Input: part model. Units: mm. Frame: model coordinates. Face numbers are marked on the shaded views. A direction names the side the tool comes from. Round coordinates to 2 decimals unless told otherwise and drop trailing zeros. Order: outer loops, then holes, each group sorted by start corner. A loop starts at its lowest first (then second) coordinate and runs counter-clockwise, first axis right, second up. Notation, with made-up numbers: (-7.5, 34) -> (35.5, 34) arc R35 ccw to (35.5, 73) -> close; hole circle Ø1 at (79, 12.5). An arc over 180 degrees is marked (long way). Use a Markdown table: item, result.
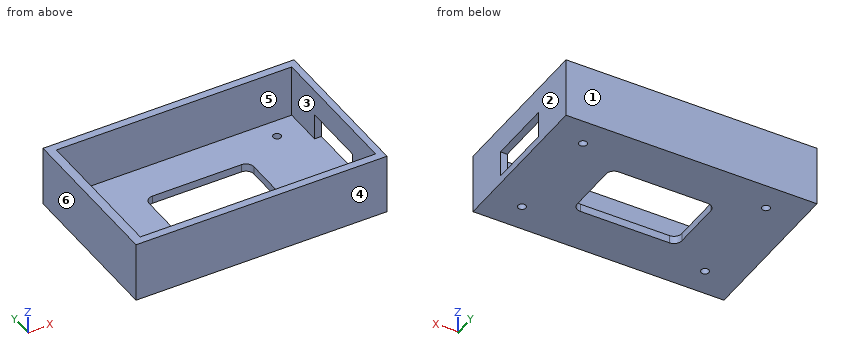
Autodesk Inventor part; units mm, degrees
ref_plane "YZ Plane" through (0, 0, 0) normal (1, 0, 0) x (0, 1, 0)
ref_plane "XZ Plane" through (0, 0, 0) normal (0, 1, 0) x (-1, 0, 0)
ref_plane "XY Plane" through (0, 0, 0) normal (0, 0, 1) x (1, 0, 0)
sketch "Sketch1" plane through (0, 0, 0) normal (0, 0, 1) x (1, 0, 0)
  line L0 (-50.0201, 33.5227) -> (45.9799, 33.5227)
  line L1 (45.9799, 33.5227) -> (45.9799, -27.4773)
  line L2 (45.9799, -27.4773) -> (-50.0201, -27.4773)
  line L3 (-50.0201, -27.4773) -> (-50.0201, 33.5227)
  line L4 (-50.0201, 33.5227) -> (-50.0201, 30.5227)
  line L5 (-46.6334, 30.5227) -> (43.3666, 30.5227)
  line L6 (43.3666, 30.5227) -> (43.3666, -24.4773)
  line L7 (43.3666, -24.4773) -> (-46.6334, -24.4773)
  line L8 (-46.6334, -24.4773) -> (-46.6334, 30.5227)
  circle A0 centre (-36.6334, 23.0227) radius 1.5
  circle A1 centre (33.3666, 23.0227) radius 1.5
  circle A2 centre (-36.6334, -16.9773) radius 1.5
  circle A3 centre (33.3666, -16.9773) radius 1.5
  line L9 (-18.6334, 15.5227) -> (15.3666, 15.5227)
  line L10 (18.3666, 12.5227) -> (18.3666, -6.4773)
  line L11 (15.3666, -9.4773) -> (-18.6334, -9.4773)
  line L12 (-21.6334, -6.4773) -> (-21.6334, 12.5227)
  arc A4 (-18.6334, 15.5227) -> (-21.6334, 12.5227) centre (-18.6334, 12.5227) ccw
  arc A5 (18.3666, 12.5227) -> (15.3666, 15.5227) centre (15.3666, 12.5227) ccw
  arc A6 (15.3666, -9.4773) -> (18.3666, -6.4773) centre (15.3666, -6.4773) ccw
  arc A7 (-21.6334, -6.4773) -> (-18.6334, -9.4773) centre (-18.6334, -6.4773) ccw
  point P0 (0, 0)
  dimension "d0" = 96
  dimension "d1" = 61
  dimension "d4" = 90
  dimension "d5" = 55
  dimension "d6" = 3
  dimension "d14" = 3
  dimension "d17" = 3
  dimension "d20" = 3
  dimension "d22" = 3
  dimension "d24" = 25
  dimension "d25" = 25
  dimension "d26" = 15
  dimension "d27" = 15
  dimension "d28" = 3
extrude "Extrusion2" add sketch "Sketch1" along normal blind 23 contours L0 L1 L2 L3
extrude "Extrusion3" add sketch "Sketch1" along normal blind 3 contours L5 L6 L7 L8
sketch "Sketch2" plane through (45.9799, -27.4773, 0) normal (1, 0, 0) x (0, 0, -1)
  line L0 (0, 0) -> (-23, 0)
  line L1 (0, 0) -> (0, 61)
  line L2 (-13, 18) -> (-3, 18)
  line L3 (-3, 18) -> (-3, 43)
  line L4 (-3, 43) -> (-13, 43)
  line L5 (-13, 43) -> (-13, 18)
  point P0 (0, 27.4773)
  dimension "d33" = 10
  dimension "d34" = 25
  dimension "d35" = 3
  dimension "d36" = 18
extrude "Extrusion4" cut sketch "Sketch2" against normal blind 3
properties part number "layer line sensor"
1) Pull-direction query (Y, two-part tool) for the marked faces 1, 2, 3 and 4; classes: +Y half, -Y half, draft (parallel to the pull), parting line (faces both ways), or undercut.
Results found:
| item | result |
|---|---|
| face 1 | +Y half |
| face 2 | draft |
| face 3 | undercut |
| face 4 | -Y half |
2) Cut plane D-D on x = -28. Return loops of the section in (y, z), and give its area (3 significant figures).
Results found:
| item | result |
|---|---|
| outline | (-27.48, 0) -> (33.52, 0) -> (33.52, 23) -> (30.52, 23) -> (30.52, 3) -> (-24.48, 3) -> (-24.48, 23) -> (-27.48, 23) -> close |
| area | 303 mm² |
3) Pin query (flat end, axial travel): pin 1 Ø0.8 at (x, y) = (44, 5.5) entering from -Z; pin 2 Ø16.5 at (x, y) = (21.5, 12.5) entering from +Z. Return the tip coordinate at first contact, or that it passes through.
Results found:
| item | result |
|---|---|
| pin 1 | stops at z = 0 |
| pin 2 | stops at z = 3 |
4) Cut plane A-A on x = -5.5. Return loops of the section in (y, z), and give its area (3 significant figures).
Results found:
| item | result |
|---|---|
| outline | (-27.48, 0) -> (-9.48, 0) -> (-9.48, 3) -> (-24.48, 3) -> (-24.48, 23) -> (-27.48, 23) -> close; (15.52, 0) -> (33.52, 0) -> (33.52, 23) -> (30.52, 23) -> (30.52, 3) -> (15.52, 3) -> close |
| area | 228 mm² |
5) Cut plane B-B on z = 16. Return loops of the section in (x, y).
Results found:
| item | result |
|---|---|
| outline | (-50.02, -27.48) -> (45.98, -27.48) -> (45.98, 33.52) -> (-50.02, 33.52) -> close; hole (-46.63, -24.48) -> (43.37, -24.48) -> (43.37, 30.52) -> (-46.63, 30.52) -> close |
6) Cut plane C-C on y = 5.5. Return loops of the section in (x, z).
Results found:
| item | result |
|---|---|
| outline | (-50.02, 0) -> (-21.63, 0) -> (-21.63, 3) -> (-46.63, 3) -> (-46.63, 23) -> (-50.02, 23) -> close; (18.37, 0) -> (45.98, 0) -> (45.98, 3) -> (18.37, 3) -> close; (43.37, 13) -> (45.98, 13) -> (45.98, 23) -> (43.37, 23) -> close |
7) Set-up query: the marked faces 5 and 6. Return all of +Z, -Z, +X, -X, +Y, -Y with unobstructed straight access to the full face (end or side cutting, diameter ignored); none if empty.
Results found:
| item | result |
|---|---|
| face 5 | +Z |
| face 6 | +Z, -Z, -X, +Y, -Y |
8) Line query: L1, parallel to Y at x = 28, z = 20.25; L2, parallel to X at y = -1.5, z = 14.5; L3, parallel to Z at x = -2, y = 23. Output: solid intervals per line, ascending. Write a range as [from, to].
Results found:
| item | result |
|---|---|
| L1 | y = [-27.48, -24.48], [30.52, 33.52] |
| L2 | x = [-50.02, -46.63], [43.37, 45.98] |
| L3 | z = [0, 3] |
